Drawing for the job (mm, zero at the part's lowest x, y, z). Give positions to 0.01 mm unless a question says otherwise; leave off trailing zeros. Loops run counter-clockwise (first coordinate to the right, second up) from the corner with the lowest first, then second, coordinate; pieces in that order, holes last. Notation, with made-up numbers: M 59,-9 L 70,-9 A17 ccw 70,6 Z; hole C 66,-26.5 d7. An arc over 180 degrees is marked long. Use CSV: the item, a comma, the result in double quotes. Start each with the question number.
(1) Slice it at A-A on x = 102. List the corners of the cut face in (y, z) (1 decimal).
(2) Slice it at C-C on z = 1.5. State how many separate pieces and enclosed holes the cut face has, and give its area (3 significant figures).
(3) Wall check: line 1 along Y through (x, z) = (105, 0.75) (1 decimal). Give the ranges that are in metal, low to high. Write a range as from..to.
(4) Flat gauge pins, fed straight in: P1, Ø1.5, axis at y = 74, z = 0.5, coming from the +X side (1 decimal); P2, Ø2.5, axis at x = 107.63, y = 107.63, coming from the -Z side; P3, Ø1.6, axis at y = 119, z = 2.5, coming from the +X side; P4, Ø1, axis at x = 2.5, z = 2.5, coming from the +Y side. Where does each tip first touch, or does it go through?
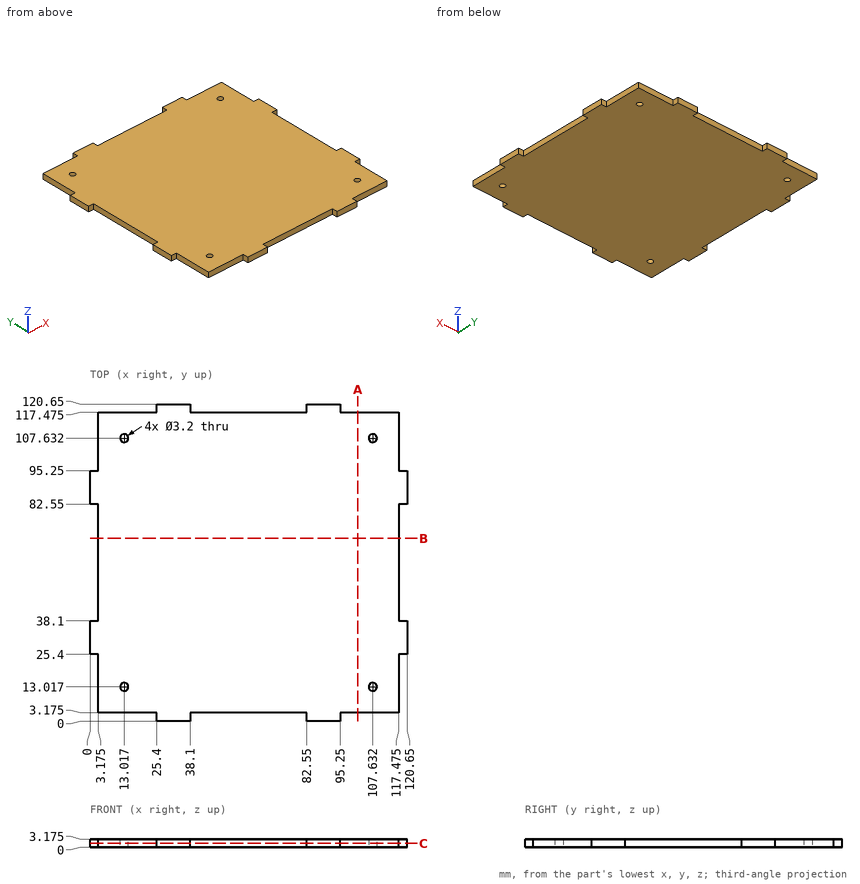
Reply:
1,outline,"M 3.2,0 L 117.5,0 L 117.5,3.2 L 3.2,3.2 Z"
2,separate pieces,"1"
2,enclosed holes,"4"
2,area,"13,400 mm^2"
3,line 1,"y = 3.2..117.5"
4,P1,"stops at x = 117.5"
4,P2,"passes through"
4,P3,"stops at x = 95.25"
4,P4,"stops at y = 95.25"
